Work out the finished part from the listing and answer in its coordinate system (mm). A direction names the side the tool comes from. Give positions to 0.01 mm unless a question says otherwise; leave off trailing zeros. Write each loop counter-clockwise with the first axis right and the second up, starting at its lowest first coordinate (ties: lowest second). Pieces come first, ordered by that corner, then holes. Notation, with made-up numbers: (25.25, -16) - (61.25, -16) arc R7 ccw to (61.25, -9) - close; hole circle Ø6 at (12, 75). An arc over 180 degrees is marked (long way). Write item = value, one per line.
from build123d import *

# Parameters (mm, degrees)
F0_R     = 6.25
F1_DEPTH = 1
F2_R     = 6.25
F2_R_2   = 5.75
F3_DEPTH = 0.75
F2_R_3   = 1
F4_DEPTH = 2


with BuildPart() as f1:
    # F0 (on Top) → F1 (new body)
    with BuildSketch(Plane.XY):
        Circle(F0_R)
    extrude(amount=F1_DEPTH)

    # F2 (on face) → F3 (join)
    with BuildSketch(Plane.XY.offset(1)):
        Circle(F2_R)
        Circle(F2_R_2, mode=Mode.SUBTRACT)
    extrude(amount=F3_DEPTH)

    # F2 (on face) → F4 (join)
    with BuildSketch(Plane.XY.offset(1)):
        Circle(F2_R_3)
    extrude(amount=F4_DEPTH)


solid = f1.part
1. Find section D-D, the plane y = 2.25. Give the vertices of the cut face in (x, z), then the cut area to 3 significant figures.
Solution:
outline = (-5.83, 0) - (5.83, 0) - (5.83, 1.75) - (5.29, 1.75) - (5.29, 1) - (-5.29, 1) - (-5.29, 1.75) - (-5.83, 1.75) - close
area = 12.5 mm^2
2. A tool of negligible diameter and unlimited length cuts with its end or side. For faces 4 (the cylindrical face through (0, -1, 2)), 5 (the flat face through (0, 0, 3)), from which of +Z, -Z, +X, -X, +Y, -Y can it reach the whole face along a straight path? Write none if from no direction.
Solution:
face_4 = +Z
face_5 = +Z, +X, -X, +Y, -Y
3. For a pull along Y with two mould halves and no side action, classify faces 1 (the flat face through (-0.1, -1.2, 1)), 2 (the cylindrical face through (5.96, 1.88, 0.86)), 3 (the flat face through (0, 0, 0)) as pulls with the +Y half, pulls with the -Y half, needs draft (parallel to the pull), parting line crosses it, or undercut.
Solution:
face_1 = undercut
face_2 = parting line crosses it
face_3 = needs draft
4. Find section C-C, the plane z = 0.5. Give the vertices of the cut face in (x, y), then the cut area to 3 significant figures.
Solution:
outline = circle Ø12.5 at (0, 0)
area = 123 mm^2
5. Straight lines are drawn through the part: line 1 (Y direction, x = 0, z = 1.6); line 2 (X direction, y = -0.25, z = 1.25) (3 decimals); line 3 (Z direction, x = 4.5, y = -4.25). For each, find the intervals that lie inside material, in ascending order.
Solution:
line_1 = -6.25 to -5.75, -1 to 1, 5.75 to 6.25
line_2 = -6.245 to -5.745, -0.968 to 0.968, 5.745 to 6.245
line_3 = 0 to 1.75
6. Find section A-A, the plane y = 0. Give the vertices of the cut face in (x, z), then the cut area to 4 significant figures.
Solution:
outline = (-6.25, 0) - (6.25, 0) - (6.25, 1.75) - (5.75, 1.75) - (5.75, 1) - (1, 1) - (1, 3) - (-1, 3) - (-1, 1) - (-5.75, 1) - (-5.75, 1.75) - (-6.25, 1.75) - close
area = 17.25 mm^2
7. Given pin 1 (1 mm diameter, centred on y = 2.5, z = 2, fed in from -X); pin 2 (1 mm diameter, centred on x = -4.5, z = 1.5, fed in from +Y); pin 3 (1.5 mm diameter, centred on x = 1.5, z = 0.5, fed in from -Y), each flat-ended and moving along its own axis, determine where each tip first touches the part or whether it passes through.
Solution:
pin_1 = -5.9
pin_2 = 4.8
pin_3 = -6.2
